Part print with two shaded views. Sizes in mm from the minimum x, y, z corner. A direction names the side the tool comes from. Give positions to 0.01 mm unless a question says otherwise; leave off trailing zeros. Write each loop counter-clockwise with the first axis right and the second up, starting at its lowest first coordinate (ties: lowest second). Pieces come first, ordered by that corner, then holes. Notation, with made-up numbers: (-29, -32) - (29, -32) arc R25 cw to (29, -20) - close; hole circle Ø1 at (17.5, 19). An arc over 180 degrees is marked (long way). One line per item, written item: value. Start each with the question number.
(1) Cut at B-B, the plane y = 28.25. List the corners of the cut face in (x, z) (1 decimal).
(2) Cut at D-D, the plane y = 15.75. List the corners of the cut face in (x, z).
(3) Probe L1, parallel to Y at x = 2, z = 1.45; L2, parallel to X at y = 28, z = 2.2; L3, parallel to Y at x = 2.9, z = 2.1 (1 decimal). List the from-to ranges inside material, lowest first.
(4) 3-axis set-ups, long thin cutter, end or side, ignore diameter. For the marked faces 4 and 5: which of +Z, -Z, +X, -X, +Y, -Y reach the whole face in a straight line?
(5) Drop a flat-ended pin along its axis: P1, Ø1.9, axis at x = 2, y = 28, coming from the -Z side. Give the stop position or say it passes through.
(6) Mould opens along Y. For the marked faces 1, 2 and 3 say: pulls with the +Y half, pulls with the -Y half, needs draft (parallel to the pull), parting line crosses it, or undercut.
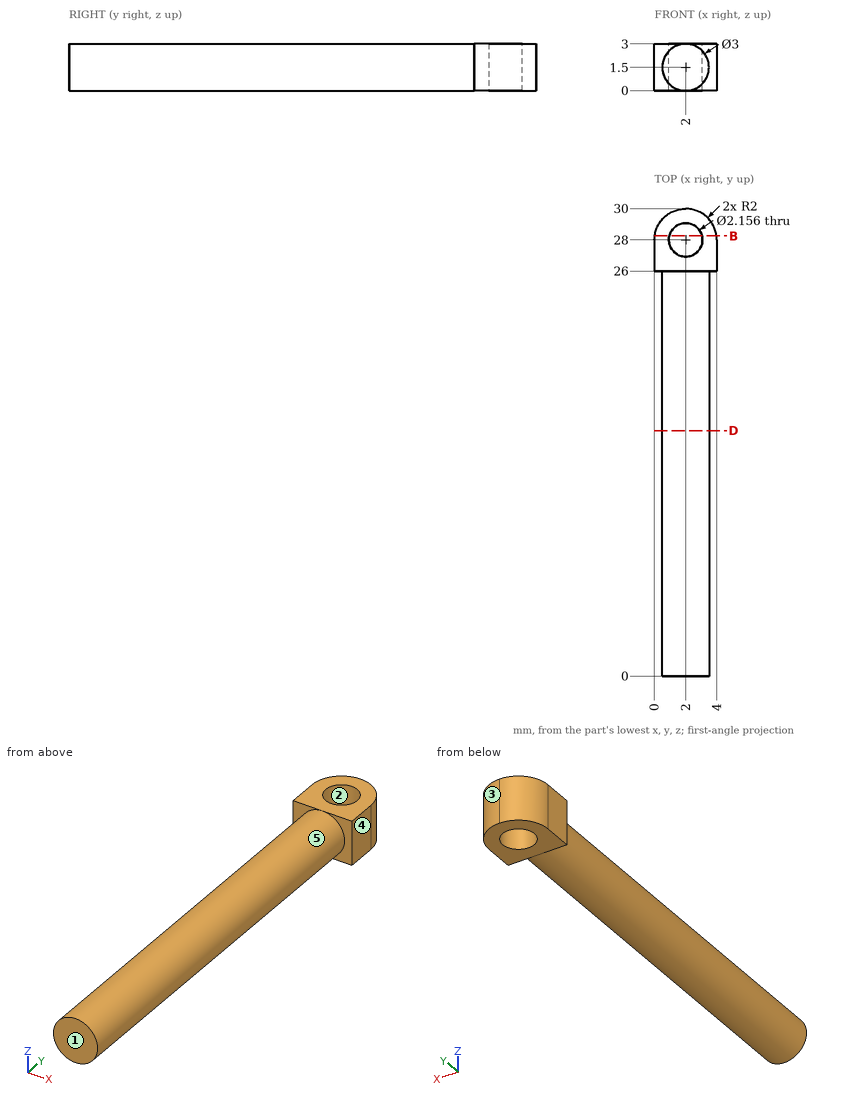
Answers follow:
1. outline: (0, 0) - (1, 0) - (1, 3) - (0, 3) - close; (3, 0) - (4, 0) - (4, 3) - (3, 3) - close
2. outline: circle Ø3 at (2, 1.5)
3. L1: y = 0 to 26.92, 29.08 to 30
3. L2: x = 0 to 0.92, 3.08 to 4
3. L3: y = 0 to 27.4, 28.6 to 29.8
4. face 4: +Z, -Z, +X, +Y, -Y
4. face 5: -Y
5. P1: passes through
6. face 1: pulls with the -Y half
6. face 2: undercut
6. face 3: pulls with the +Y half
